Verification items for the finished model (mm, model axes). Face numbers are marked on the shaded views. A direction names the side the tool comes from. Give positions to 0.01 mm unless a question says otherwise; leave off trailing zeros. Write each loop counter-clockwise with the first axis right and the second up, starting at its lowest first coordinate (ties: lowest second). Pieces come first, ordered by that corner, then holes. Notation, with made-up numbers: (28.25, -24) -> (50.25, -24) arc R23 cw to (50.25, 11) -> close; hole circle Ø9 at (60, 23.5). An arc over 180 degrees is marked (long way). Answer as CSV lines item,"result". Start each with the question number.
1) Material ranges on L1, parallel to X at y = -50, z = 5.5; L2, parallel to X at y = -18, z = 3; L3, parallel to X at y = -19, z = 5, recorded low to high.
2) Gauge pin test, flat ends, axial feed: pin 1 Ø6 at (x, z) = (-19, 2) entering from -Y; pin 2 Ø2 at (x, y) = (-33, -131.94) entering from -Z; pin 3 Ø3 at (x, y) = (-33, -50) entering from +Z; pin 4 Ø2.5 at (x, z) = (-4, 5) entering from +Y. Record the tip position at first contact, or that the pin passes through.
3) Sectioned sample at C-C on x = -45. Record the cut outline in (y, z).
4) Mould release check, pull along X, two halves, no side actions. Record for the marked faces 4, 5, 6 and 7: released by +X, released by -X, zero draft, split by the parting line, or undercut.
5) Tool access check on the marked faces 1, 2 and 3. Record the directions out of +Z, -Z, +X, -X, +Y, -Y that give a thin tool (end or side, any length) a straight path to the whole face; none if there is none.
6) Sectioned sample at A-A on z = 2.5. Record the cut outline in (x, y).
7) Sectioned sample at B-B on x = -62. Record the cut outline in (y, z), and give its area (3 significant figures).
```python
from build123d import *

# Parameters (mm, degrees)
F1_DEPTH     = 10
F3_DEPTH     = 9
F5_D         = 2.4
F6_T1_DEPTH  = 55
F6_T3_DEPTH  = 5
F6_T9_DEPTH  = 64.75
F6_T13_DEPTH = 14.75
F6_T16_DEPTH = 24.5
F6_T18_DEPTH = 74.5


# Not quite as in the source:
# - a fillet or chamfer that OpenCascade refuses, or shapes differently, is made with other operations: its cross-section is extruded or revolved along the edge and cut away or added
# - a feature names something its author has since deleted; it is built from what else it names


with BuildPart() as f1:
    # F0 (on Top) → F1 (new body)
    with BuildSketch(Plane.XY):
        with BuildLine():
            Line((-30, 0), (-70, 0))
            Line((-70, 0), (-70, -100))
            ThreePointArc((-70, -100), (-59.7487373415, -124.7487373415), (-35, -135))
            Line((-35, -135), (-30, -135))
            Line((-30, -135), (-30, -42))
            ThreePointArc((-30, -42), (-28.5355339059, -38.4644660941), (-25, -37))
            Line((-25, -37), (-15, -37))
            ThreePointArc((-15, -37), (-4.9050660078, -31.4878584828), (-4.0842494776, -20.0153846154))
            ThreePointArc((-4.0842494776, -20.0153846154), (-4.0158481001, -19.0593451264), (-3.1746036007, -18.6))
            Line((-3.1746036007, -18.6), (-1, -18.6))
            ThreePointArc((-1, -18.6), (-0.2928932188, -18.3071067812), (0, -17.6))
            ThreePointArc((0, -17.6), (-0.2928932188, -16.8928932188), (-1, -16.6))
            Line((-1, -16.6), (-6.3162509151, -16.6))
            ThreePointArc((-6.3162509151, -16.6), (-7.0233576963, -16.8928932188), (-7.3162509151, -17.6))
            Line((-7.3162509151, -17.6), (-7.3162509151, -18.2477780079))
            ThreePointArc((-7.3162509151, -18.2477780079), (-7.2621451309, -18.5722531726), (-7.1056826501, -18.8616163708))
            ThreePointArc((-7.1056826501, -18.8616163708), (-14.7582290616, -34.9970769134), (-23.1818181818, -19.2504042542))
            ThreePointArc((-23.1818181818, -19.2504042542), (-23.0465374108, -18.9769560242), (-23, -18.6754446797))
            ThreePointArc((-23, -18.6754446797), (-23.6984886554, -17.7219820904), (-24.8181818182, -18.1004851051))
            ThreePointArc((-24.8181818182, -18.1004851051), (-26.2938104102, -20.9441589751), (-26.9644443663, -24.0769230769))
            ThreePointArc((-26.9644443663, -24.0769230769), (-27.2821151763, -24.7337993857), (-27.9614813968, -25))
            Line((-27.9614813968, -25), (-29, -25))
            ThreePointArc((-29, -25), (-29.7071067812, -24.7071067812), (-30, -24))
            Line((-30, -24), (-30, 0))
        make_face()
    extrude(amount=F1_DEPTH)

    # F2 (on face) → F3 (cut)
    with BuildSketch(Plane.XY.offset(10)):
        with BuildLine():
            Line((-35, -55), (-35, 0))
            Line((-35, 0), (-70, 0))
            Line((-70, 0), (-70, -100))
            ThreePointArc((-70, -100), (-59.7487373415, -124.7487373415), (-35, -135))
            Line((-35, -135), (-30, -135))
            Line((-30, -135), (-30, -55))
            Line((-30, -55), (-35, -55))
        make_face()
    extrude(amount=-F3_DEPTH, mode=Mode.SUBTRACT)

    # F5 (through all)
    with Locations(Plane.XY.offset(10)):
        with Locations((-67, -3), (-50, -128.2665880502), (-33, -131.9374388453), (-33, -85), (-33, -50), (-33, -3), (-67, -95)):
            Hole(F5_D / 2)

    # F6: fillet of radius 3.9 on 4 edges, made by hand

    # F6_s2 → F6_t1 (join)
    with BuildSketch(Plane.XZ):
        with BuildLine():
            ThreePointArc((-35, 4.9), (-36.1422835534, 2.1422835534), (-38.9, 1))
            Line((-38.9, 1), (-35, 1))
            Line((-35, 1), (-35, 4.9))
        make_face()
    extrude(amount=F6_T1_DEPTH)

    # F6_s4 → F6_t3 (join)
    with BuildSketch(Plane.YZ.offset(-35)):
        with BuildLine():
            ThreePointArc((-55, 4.9), (-56.1422835534, 2.1422835534), (-58.9, 1))
            Line((-58.9, 1), (-55, 1))
            Line((-55, 1), (-55, 4.9))
        make_face()
    extrude(amount=F6_T3_DEPTH)


with BuildPart() as f6_tool7:
    # F6_s8 → F6_t9 (new body)
    with BuildSketch(Plane.XZ.offset(64.75)):
        with BuildLine():
            ThreePointArc((-35, 4.9), (-36.1422835534, 2.1422835534), (-38.9, 1))
            Line((-38.9, 1), (-35, 1))
            Line((-35, 1), (-35, 4.9))
        make_face()
    extrude(amount=-F6_T9_DEPTH)

    split(bisect_by=Plane.XZ.offset(55), keep=Keep.TOP)


with BuildPart() as f6_tool11:
    # F6_s12 → F6_t13 (new body)
    with BuildSketch(Plane.YZ.offset(-30)):
        with BuildLine():
            ThreePointArc((-55, 4.9), (-56.1422835534, 2.1422835534), (-58.9, 1))
            Line((-58.9, 1), (-55, 1))
            Line((-55, 1), (-55, 4.9))
        make_face()
    extrude(amount=-F6_T13_DEPTH)

    split(bisect_by=Plane.YZ.offset(-35), keep=Keep.BOTTOM)


with BuildPart() as f6_tool7_1:
    add(f6_tool7.part)

    # F6_t15: intersect F6_tool11
    add(f6_tool11.part, mode=Mode.INTERSECT)


with BuildPart() as f1_1:
    add(f1.part)

    # F6_t5: union F6_tool7
    add(f6_tool7_1.part)

    # F6_s17 → F6_t16 (cut)
    with BuildSketch(Plane.YZ.offset(-44.75)):
        with BuildLine():
            ThreePointArc((-55, 6.1), (-53.8577164466, 8.8577164466), (-51.1, 10))
            Line((-51.1, 10), (-55, 10))
            Line((-55, 10), (-55, 6.1))
        make_face()
    extrude(amount=F6_T16_DEPTH, mode=Mode.SUBTRACT)

    # F6_s19 → F6_t18 (cut)
    with BuildSketch(Plane.XZ.offset(-9.75)):
        with BuildLine():
            ThreePointArc((-35, 6.1), (-33.8577164466, 8.8577164466), (-31.1, 10))
            Line((-31.1, 10), (-35, 10))
            Line((-35, 10), (-35, 6.1))
        make_face()
    extrude(amount=F6_T18_DEPTH, mode=Mode.SUBTRACT)


solid = f1_1.part
```
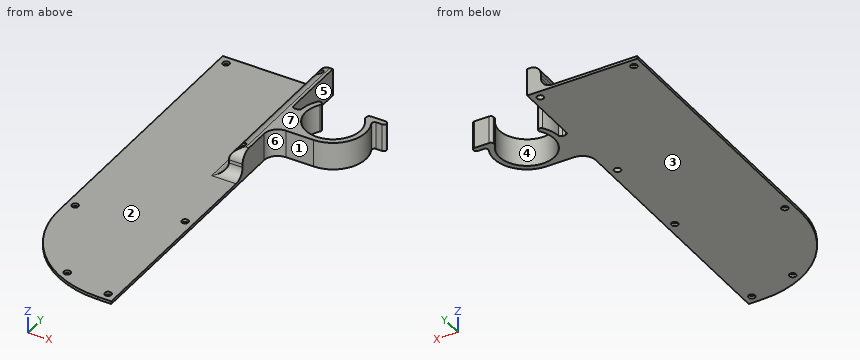
Ans:
1,L1,"x = -35 to -34.2, -31.8 to -30"
1,L2,"x = -35.49 to -30, -24.74 to -23.26, -7.32 to -0.08"
1,L3,"x = -35 to -30, -25.39 to -23.05, -7 to -3.97"
2,pin 1,"stops at y = -37"
2,pin 2,"passes through"
2,pin 3,"stops at z = 9.98"
2,pin 4,"stops at y = -16.6"
3,outline,"(-133.54, 0) -> (0, 0) -> (0, 1) -> (-133.54, 1) -> close"
4,face 4,"undercut"
4,face 5,"undercut"
4,face 6,"released by +X"
4,face 7,"zero draft"
5,face 1,"+Z, -Z, +X, -Y"
5,face 2,"+Z, -X, -Y"
5,face 3,"-Z, +X, -X, +Y, -Y"
6,outline,"(-35.83, -55.83) -> (-30, -55.83) -> (-30, -42) arc R5 cw to (-25, -37) -> (-15, -37) arc R12 ccw to (-4.08, -20.02) arc R1 cw to (-3.17, -18.6) -> (-1, -18.6) arc R1 ccw to (-1, -16.6) -> (-6.32, -16.6) arc R1 ccw to (-7.32, -17.6) -> (-7.32, -18.25) arc R1 ccw to (-7.11, -18.86) arc R10 cw (long way) to (-23.18, -19.25) arc R1 ccw to (-24.82, -18.1) arc R12 ccw to (-26.96, -24.08) arc R1 cw to (-27.96, -25) -> (-29, -25) arc R1 cw to (-30, -24) -> (-30, 0) -> (-35.83, 0) -> close; hole circle Ø2.4 at (-33, -50); hole circle Ø2.4 at (-33, -3)"
7,outline,"(-122.27, 0) -> (0, 0) -> (0, 1) -> (-122.27, 1) -> close"
7,area,"122 mm²"
